Can you work these out from the model? Positions are in its coordinate system, mm. A direction names the side the tool comes from. Give positions to 0.01 mm unless a question says otherwise; leave off trailing zeros. Loops run counter-clockwise (first coordinate to the right, second up) from the corner with the lowest first, then second, coordinate; pieces in that order, holes last. Notation, with made-up numbers: (-35, 65) -> (-17, 65) arc R18 cw to (-17, 85) -> close; hole circle Ø1 at (34, 4). An arc over 180 degrees is marked (long way). Return JSON: item names as keys, results as strings. Group by question number.
Q1. Thinking about a two-plate mould opening in X: for faces 3 (the flat face through (3, 0, -3)), 4 (the cylindrical face through (3.755, 14.79, 11.923)), 5 (the cylindrical face through (-0.867, 7.3, 3.905)), which applies, pulls with the +X half, pulls with the -X half, needs draft (parallel to the pull), parting line crosses it, or undercut?
Q2. Which directions (+Z, -Z, +X, -X, +Y, -Y) give clear straight access to the entire face, cutting with the end or side of a thin tool? Please do faces 1 (the flat face through (-5.4, 30, -0.2)), 2 (the cylindrical face through (1.08, 22.4, 4.88)).
Q3. Suppose I cut it at C-C, the plane y = 12. Please give me the cut outline in (x, z).
Q4. I need wall thicknesses on line 1 along X through (y, z) = (15.75, -4); line 2 along Z through (x, y) = (9, 4). Which ranges of each line are inside material? Lowest first, please. Write a range as [from, to].
Q5. Suppose I cut it at B-B, the plane x = 0. Please give me the cut outline in (y, z).
Q6. Suppose I cut it at D-D, the plane x = 9.75. Please give me the cut outline in (y, z), and give its area (3 significant figures).
Q7. Suppose I cut it at A-A, the plane z = 0. Please give me the cut outline in (x, y).
Q8. Will these pins go through, and if not, where does the flat tip stop? pin 1 (1.5 mm diameter, centred on x = -2.5, z = 3.5, fed in from -Y); pin 2 (5 mm diameter, centred on y = 18, z = 7, fed in from -X); pin 3 (2 mm diameter, centred on y = 10.5, z = 2, fed in from -X).
```python
from build123d import *

# Parameters (mm, degrees)
SKETCH1_R                      = 12.5
BOSS_EXTRUDE1_DEPTH            = 30
F_10_0_10_DIAMETER_HOLE1_D     = 10
F_10_0_10_DIAMETER_HOLE1_DEPTH = 15
F_10_0_10_DIAMETER_HOLE1_TIP   = 3.004303095
F_8_0_8_DIAMETER_HOLE1_D       = 8
F_8_0_8_DIAMETER_HOLE1_DEPTH   = 15
F_8_0_8_DIAMETER_HOLE1_TIP     = 2.403442476


with BuildPart() as part:
    # Sketch1 → Boss-Extrude1 (new body)
    with BuildSketch(Plane(origin=(0, 0, 0), x_dir=(1, 0, 0), z_dir=(0, 1, 0))):
        with Locations(Location((0, 0, 0), (0, 0, 270))):
            Circle(SKETCH1_R)
    extrude(amount=BOSS_EXTRUDE1_DEPTH)

    # Ø10.0 (10) Diameter Hole1
    with Locations(Plane(origin=(0, 30, 0), x_dir=(1, 0, 0), z_dir=(0, 1, 0))):
        with Locations((0, 0)):
            Hole(F_10_0_10_DIAMETER_HOLE1_D / 2, depth=F_10_0_10_DIAMETER_HOLE1_DEPTH)
            with Locations((0, 0, -(F_10_0_10_DIAMETER_HOLE1_DEPTH + F_10_0_10_DIAMETER_HOLE1_TIP / 2))):  # 118° drill point
                Cone(0, F_10_0_10_DIAMETER_HOLE1_D / 2, F_10_0_10_DIAMETER_HOLE1_TIP, mode=Mode.SUBTRACT)

    # Ø8.0 (8) Diameter Hole1
    with Locations(Plane(origin=(0, 0, 0), x_dir=(-1, 0, 0), z_dir=(0, -1, 0))):
        with Locations((0, 0)):
            Hole(F_8_0_8_DIAMETER_HOLE1_D / 2, depth=F_8_0_8_DIAMETER_HOLE1_DEPTH)
            with Locations((0, 0, -(F_8_0_8_DIAMETER_HOLE1_DEPTH + F_8_0_8_DIAMETER_HOLE1_TIP / 2))):  # 118° drill point
                Cone(0, F_8_0_8_DIAMETER_HOLE1_D / 2, F_8_0_8_DIAMETER_HOLE1_TIP, mode=Mode.SUBTRACT)


solid = part.part
```
Ans:
{
 "1": {"face 3": "needs draft", "face 4": "parting line crosses it", "face 5": "undercut"},
 "2": {"face 1": "+Z, -Z, +X, -X, +Y", "face 2": "+Y"},
 "3": {"outline": "circle Ø25 at (0, 0); hole circle Ø8 at (0, 0)"},
 "4": {"line 1": "x = [-11.84, -3], [3, 11.84]", "line 2": "z = [-8.67, 8.67]"},
 "5": {"outline": "(0, -12.5) -> (30, -12.5) -> (30, -5) -> (15, -5) -> (14.4, -4) -> (0, -4) -> close; (0, 4) -> (14.4, 4) -> (15, 5) -> (30, 5) -> (30, 12.5) -> (0, 12.5) -> close"},
 "6": {"outline": "(0, -7.82) -> (30, -7.82) -> (30, 7.82) -> (0, 7.82) -> close", "area": "469 mm^2"},
 "7": {"outline": "(-12.5, 0) -> (-4, 0) -> (-4, 14.4) -> (-5, 15) -> (-5, 30) -> (-12.5, 30) -> close; (4, 0) -> (12.5, 0) -> (12.5, 30) -> (5, 30) -> (5, 15) -> (4, 14.4) -> close"},
 "8": {"pin 1": "stops at y = 0", "pin 2": "stops at x = -11.66", "pin 3": "stops at x = -12.46"}
}
